from build123d import *

# Parameters (mm, degrees)
F2_R = 3.175


with BuildPart() as f3:
    # F3: sweep along a path in F0
    with BuildLine(Plane.XZ) as f3_path:
        Line((-50.8, -126.1922290944), (-50.8, -138.8922290944))
        ThreePointArc((-50.8, -138.8922290944), (-47.0802561211, -147.8724852155), (-38.1, -151.5922290944))
        ThreePointArc((-38.1, -151.5922290944), (-29.1197438789, -147.8724852155), (-25.4, -138.8922290944))
        Line((-25.4, -138.8922290944), (-25.4, 140.5077709056))
        ThreePointArc((-25.4, 140.5077709056), (-21.6802561211, 149.4880270267), (-12.7, 153.2077709056))
        ThreePointArc((-12.7, 153.2077709056), (-3.7197438789, 149.4880270267), (0, 140.5077709056))
        Line((0, 140.5077709056), (0, 127.8077709056))
    # F2 (on plane+point) → F3 (sweep)
    with BuildSketch(Plane.XY.offset(-126.1922290944)):
        with Locations((-50.8, 0)):
            Circle(F2_R)
    sweep(path=f3_path.line)


solid = f3.part
Can you work these out from the model? Positions are in its coordinate system, mm. A direction names the side the tool comes from. Give positions to 0.01 mm unless a question says otherwise; leave off trailing zeros. Order: outer loops, then holes, each group sorted by start corner. A loop starts at its lowest first (then second) coordinate and runs counter-clockwise, first axis right, second up. Notation, with made-up numbers: M 27.5,-22 L 63.5,-22 A12 ccw 63.5,-15 Z; hole C 38,15 d8. An arc over 180 degrees is marked long. Use one line per item in the form item = value. Start each with the question number.
Item 1: We'd pull the mould along X, two halves only. Please class faces 4 (the flat face through (-51, 0, -126.192)), 5 (the cylindrical face through (-53.97, -0.14, -132.63)): +X half, -X half, draft (parallel to the pull), parting line (faces both ways), or undercut.
Item 2: Will these pins go through, and if not, where does the flat tip stop? pin 1 Ø1.9 at (x, y) = (-51.5, 0) entering from +Z; pin 2 Ø1.5 at (x, z) = (-28.5, 111.5) entering from -Y (3 decimals); pin 3 Ø1 at (y, z) = (-1.5, -75) entering from +X.
Item 3: If we section it at B-B (y = -1.75): Write out the boundary of the cut face in (x, z), then the cut area to 3 significant figures.
Item 4: If I drill on line 1 along X through (y, z) = (-0.25, -64.5); line 2 along X through (y, z) = (0.5, 45.5); line 3 along Y through (x, z) = (-25, 112.5), over which ranges is the centre line in solid material (lowest first)?
Item 5: If we section it at A-A (z = 133.5): Write out the boundary of the cut face in (x, y) (3 decimals).
Item 6: For faces 1 (the flat face through (0, 0, 127.808)), 2 (the cylindrical face through (-0.69, 3.1, 134.07)), 3 (the cylindrical face through (-28.43, -0.95, 2.76)), which set-ups out of +Z, -Z, +X, -X, +Y, -Y let a thin tool reach every point of the face, with its end or its side?
Item 7: If we section it at C-C (z = 68): Write out the boundary of the cut face in (x, y) (3 decimals), then the cut area to 3 significant figures.
Outcome:
q1.face_4 = draft
q1.face_5 = undercut
q2.pin_1 = -126.19
q2.pin_2 = -2.135
q2.pin_3 = -22.39
q3.outline = M -53.45,-138.89 A15.35 ccw -22.75,-138.89 L -22.75,140.51 A10.05 cw -2.65,140.51 L -2.65,127.81 L 2.65,127.81 L 2.65,140.51 A15.35 ccw -28.05,140.51 L -28.05,-138.89 A10.05 cw -48.15,-138.89 L -48.15,-126.19 L -53.45,-126.19 Z
q3.area = 2,040 mm2
q4.line_1 = -28.57 to -22.23
q4.line_2 = -28.54 to -22.26
q4.line_3 = -3.15 to 3.15
q5.outline = C -25.4,0 d6.35; C 0,0 d6.35
q6.face_1 = -Z, +X, +Y, -Y
q6.face_2 = -Z
q6.face_3 = none
q7.outline = C -25.4,0 d6.35
q7.area = 31.7 mm2
